Check sheet for the modelled part. Datum: model origin and axes. Units: mm. A direction names the side the tool comes from. Give positions to 0.01 mm unless a question says otherwise; leave off trailing zeros. Write each loop counter-clockwise with the first axis right and the second up, starting at its lowest first coordinate (ties: lowest second). Pieces come first, ordered by that corner, then holes. Notation, with made-up numbers: (5, 20.5) -> (31, 20.5) arc R29 ccw to (31, 43.5) -> close; hole circle Ø11 at (46.25, 10.5). An arc over 180 degrees is marked (long way). Return JSON: item names as keys, results as strings.
from build123d import *

# Parameters (mm, degrees)
SKETCH1_W           = 1.6
SKETCH1_H           = 15
BOSS_EXTRUDE1_DEPTH = 36
SKETCH2_R           = 2.5
BOSS_EXTRUDE2_DEPTH = 5.8
SKETCH3_W           = 7
SKETCH3_H           = 6
BOSS_EXTRUDE3_DEPTH = 7


with BuildPart() as part:
    # Sketch1 → Boss-Extrude1 (new body)
    with BuildSketch(Plane.XY.offset(7)):
        with Locations((15, -121)):
            Rectangle(SKETCH1_W, SKETCH1_H)
    extrude(amount=BOSS_EXTRUDE1_DEPTH)

    # Sketch2 → Boss-Extrude2 (add)
    with BuildSketch(Plane.XY.offset(43)):
        with Locations(Location((15, -119, 0), (0, 0, 108.662924885))):
            Circle(SKETCH2_R)
    extrude(amount=BOSS_EXTRUDE2_DEPTH)

    # Sketch3 → Boss-Extrude3 (add)
    with BuildSketch(Plane.XY.offset(18)):
        with Locations((10.7, -117.5)):
            Rectangle(SKETCH3_W, SKETCH3_H)
    extrude(amount=BOSS_EXTRUDE3_DEPTH)


solid = part.part
(1) Cross-section at B-B on x = 15. Enter the section's corners in (y, z), then the cut area to 3 significant figures.
Reply:
{"outline": "(-128.5, 7) -> (-113.5, 7) -> (-113.5, 43) -> (-116.5, 43) -> (-116.5, 48.8) -> (-121.5, 48.8) -> (-121.5, 43) -> (-128.5, 43) -> close", "area": "569 mm^2"}
(2) Release check for a two-part mould opening along Z. For faces 1 (the flat face through (15, -125, 43)), 2 (the flat face through (13, -119, 43)), 3 (the flat face through (15.8, -121, 25)) record: pulls with the +Z half, pulls with the -Z half, needs draft (parallel to the pull), parting line crosses it, or undercut.
Reply:
{"face 1": "pulls with the +Z half", "face 2": "undercut", "face 3": "needs draft"}
(3) Cross-section at A-A on z = 20. Enter the section's corners in (x, y).
Reply:
{"outline": "(7.2, -120.5) -> (14.2, -120.5) -> (14.2, -128.5) -> (15.8, -128.5) -> (15.8, -113.5) -> (14.2, -113.5) -> (14.2, -114.5) -> (7.2, -114.5) -> close"}
(4) Set-up check for faces 4 (the flat face through (11, -117, 18)), 5 (the cylindrical face through (15.7, -121.4, 45.9)), 6 (the flat face through (17, -119, 43)), 7 (the flat face through (11, -114.5, 21)): record each of +Z, -Z, +X, -X, +Y, -Y from which the full face is reachable in a straight line by a thin tool's end or side.
Reply:
{"face 4": "-Z, -X, +Y, -Y", "face 5": "+Z", "face 6": "-Z, +X, +Y, -Y", "face 7": "+Z, -Z, -X, +Y"}
(5) Depth check by flat-ended pin: pin 1 Ø0.8 at (x, y) = (14.5, -115) entering from +Z; pin 2 Ø0.9 at (x, y) = (13, -119) entering from -Z; pin 3 Ø4 at (x, z) = (10.5, 41.5) entering from -Y; pin 4 Ø4 at (y, z) = (-116, 37) entering from +X. Enter the tip coordinate at first touch or a pass-through.
Reply:
{"pin 1": "z = 43", "pin 2": "z = 18", "pin 3": "through", "pin 4": "x = 15.8"}
(6) Thickness scan on L1, parallel to X at y = -114.75, z = 35.5; L2, parallel to Z at x = 12.75, y = -119.25; L3, parallel to Y at x = 13.5, z = 21. Record the ranges inside material, lowest first.
Reply:
{"L1": "14.2 to 15.8", "L2": "18 to 25, 43 to 48.8", "L3": "-120.5 to -114.5"}
(7) Cross-section at C-C on y = -119. Enter the section's corners in (x, z), then the cut area to 3 significant figures.
Reply:
{"outline": "(7.2, 18) -> (14.2, 18) -> (14.2, 7) -> (15.8, 7) -> (15.8, 43) -> (17.5, 43) -> (17.5, 48.8) -> (12.5, 48.8) -> (12.5, 43) -> (14.2, 43) -> (14.2, 25) -> (7.2, 25) -> close", "area": "136 mm^2"}
(8) Cross-section at D-D on z = 45.5. Enter the section's corners in (x, y).
Reply:
{"outline": "circle Ø5 at (15, -119)"}
